Solid Edge part; units mm, degrees
sketch "Sketch1" plane through (0, 0, 0) normal (0, -1, 0) x (1, 0, 0)
  line L0 (3, 12) -> (3, 0)
  line L1 (3, 0) -> (11, 0)
  line L2 (11, 0) -> (11, 2)
  line L3 (11, 2) -> (5, 2)
  line L4 (5, 2) -> (5, 12)
  line L5 (5, 12) -> (3, 12)
  dimension "D1" = 3
  dimension "D2" = 11
revolve "RevolvedProtrusion1" add sketch "Sketch1" angle 360 about axis through (0, 0, 54) along (0, 0, -1)
hole "Hole1" at (8, 0, 2) direction (0, 0, -1) diameter 2.9 end up to next
pattern_circular "Pattern1" count 4 over 360 about axis through (0, 0, 2) along (0, 0, 1) of "Hole1"
chamfer "Chamfer_1" distance 0.5 angle 30 2 edges at (-3, 0, 12) (-3, 0, 0) measured on face at (1.6602, -2.4988, 9.88)
properties material "Stainless steel"
Source: CAD feature listing. Evaluate the final solid. Frame: model axes, mm. A direction names the side the tool comes from. Round coordinates to 2 decimals unless told otherwise and drop trailing zeros. Loops run counter-clockwise (first coordinate to the right, second up) from the corner with the lowest first, then second, coordinate; pieces in that order, holes last. Notation, with made-up numbers: M 35.5,4 L 59.5,4 A12 cw 59.5,12 Z; hole C 61.5,68 d3. An arc over 180 degrees is marked long. Use a Markdown table: item, result. Add a question column.
1. Section query D-D on z = 9.5. Return the cut outline in (x, y).
2. Reachability of faces 1 (the cylindrical face through (-3, 0, 6)), 2 (the flat face through (2, 5, 2)) from +Z, -Z, +X, -X, +Y, -Y: full face, straight path, thin tool, end or side. Return the list, or none.
3. Contact query for flat-ended pins moving along their axis: P1, Ø1, axis at x = -1.5, y = -8.5, coming from the +Z side; P2, Ø4, axis at y = 8.5, z = 7.5, coming from the -X side; P3, Ø1, axis at y = -8, z = 2, coming from the +X side; P4, Ø5, axis at x = 4, z = 7.5, coming from the +Y side. Output: stop coordinate, or through.
4. Section query A-A on y = 0. Return the cut outline in (x, z).
5. Section query C-C on y = 8. Return the cut outline in (x, z), then the cut area to 3 significant figures.
6. Line query: line 1 (Y direction, x = 0, z = 1.1); line 2 (Z direction, x = -10, y = -1.5); line 3 (Y direction, x = 0, z = 9). Output: solid intervals per line, ascending.
7. Mould query, pull axis Y, two halves, no side actions, for faces 3 (the cylindrical face through (-1.08, -4.88, 7.07)), 4 (the flat face through (2, -3, 0)), 5 (the cylindrical face through (-0.314, 6.584, 1.014)). Classes: pulls with the +Y half, pulls with the -Y half, needs draft (parallel to the pull), parting line crosses it, or undercut.
Reported:
| question | item | result |
|---|---|---|
| 1 | outline | C 0,0 d10; hole C 0,0 d6 |
| 2 | face 1 | +Z, -Z |
| 2 | face 2 | +Z |
| 3 | P1 | stops at z = 2 |
| 3 | P2 | passes through |
| 3 | P3 | stops at x = 8.05 |
| 3 | P4 | stops at y = 4.77 |
| 4 | outline | M -11,0 L -9.45,0 L -9.45,2 L -11,2 Z; M -6.55,0 L -3.29,0 L -3,0.5 L -3,11.5 L -3.29,12 L -5,12 L -5,2 L -6.55,2 Z; M 3,0.5 L 3.29,0 L 6.55,0 L 6.55,2 L 5,2 L 5,12 L 3.29,12 L 3,11.5 Z; M 9.45,0 L 11,0 L 11,2 L 9.45,2 Z |
| 5 | outline | M -7.55,0 L -1.45,0 L -1.45,2 L -7.55,2 Z; M 1.45,0 L 7.55,0 L 7.55,2 L 1.45,2 Z |
| 5 | area | 24.4 mm² |
| 6 | line 1 | y = -11 to -9.45, -6.55 to -3, 3 to 6.55, 9.45 to 11 |
| 6 | line 2 | z = 0 to 2 |
| 6 | line 3 | y = -5 to -3, 3 to 5 |
| 7 | face 3 | parting line crosses it |
| 7 | face 4 | needs draft |
| 7 | face 5 | undercut |
